Can you work these out from the drawing? Everything is in mm from the part's minimum corner. Give positions to 0.01 mm unless a question says otherwise; leave off trailing zeros. Order: outer loops, then holes, each group sorted by start corner. A loop starts at its lowest first (then second) coordinate and runs counter-clockwise, first axis right, second up. Notation, with made-up numbers: (-7, -4) - (39, -4) arc R20 cw to (39, 18) - close; hole circle Ø3 at (0.5, -27.5). An arc over 180 degrees is marked (long way). Answer as a JSON object with one key per item and string values.
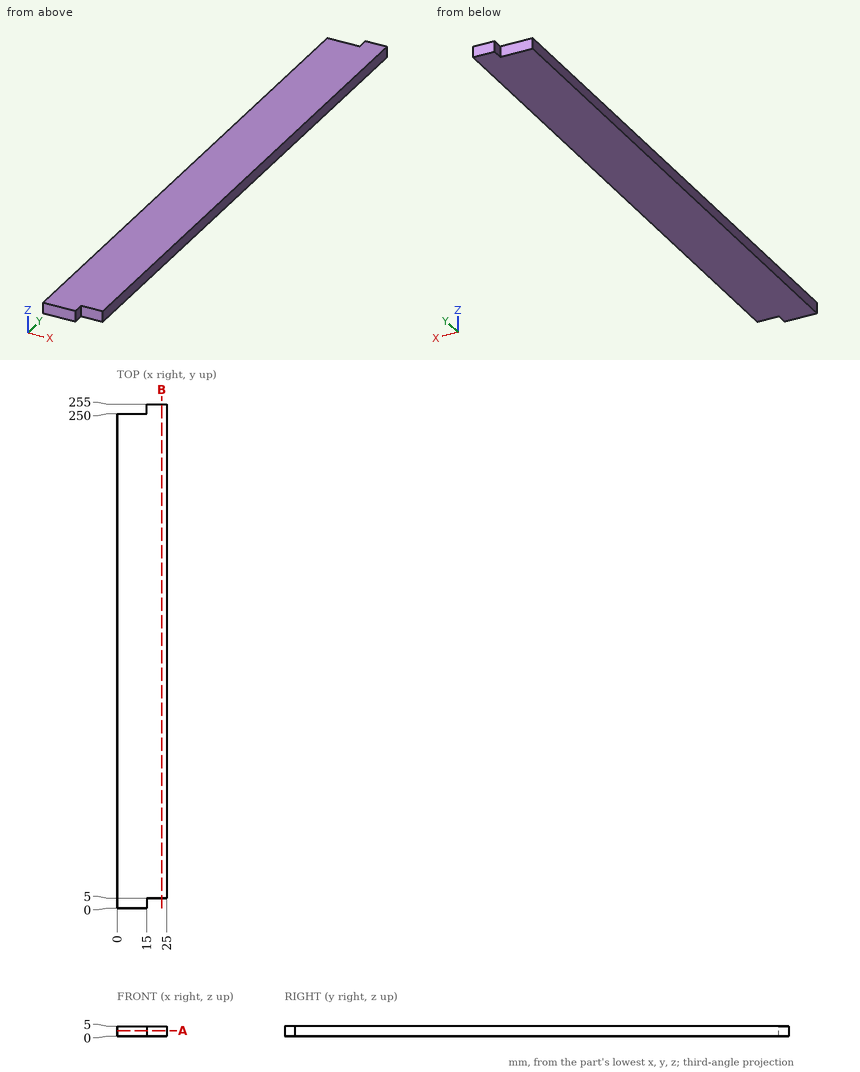
Q1. I need wall thicknesses on L1, parallel to Y at x = 6.5, z = 3.65; L2, parallel to Y at x = 20.25, z = 1.5. Which ranges of each line are inside material? Lowest first, please.
Recorded:
{"L1": "y = 0 to 250", "L2": "y = 5 to 255"}
Q2. If we section it at B-B, the plane x = 22.5: Please give me the cut outline in (y, z), then the cut area to 3 significant figures.
Recorded:
{"outline": "(5, 0) - (255, 0) - (255, 5) - (5, 5) - close", "area": "1,250 mm^2"}
Q3. If we section it at A-A, the plane z = 2.75: Please give me the cut outline in (x, y).
Recorded:
{"outline": "(0, 0) - (15, 0) - (15, 5) - (25, 5) - (25, 255) - (15, 255) - (15, 250) - (0, 250) - close"}
Q4. I'm going to push flat-ended pins straight in: pin 1 Ø1.5 at (x, z) = (9, 1.5) entering from +Y; pin 2 Ø1.5 at (y, z) = (252.5, 1.5) entering from -X; pin 3 Ø2.5 at (y, z) = (2, 1.5) entering from +X. Where does each tip first touch, or does it pass through?
Recorded:
{"pin 1": "stops at y = 250", "pin 2": "stops at x = 15", "pin 3": "stops at x = 15"}
